```python
from build123d import *

# Parameters (mm, degrees)
SKETCH_W        = 130
SKETCH_H        = 200
PAD_DEPTH       = 2.5
SKETCH001_R     = 2.5
POCKET_DEPTH    = 5.001
SKETCH002_W     = 10
SKETCH002_H     = 5
POCKET001_DEPTH = 5.001
SKETCH003_W     = 5
SKETCH003_H     = 10
PAD001_DEPTH    = 5
SKETCH004_W     = 10
SKETCH004_H     = 5
PAD002_DEPTH    = 5
FILLET_R        = 7


with BuildPart() as part:
    # Sketch → Pad (new body, symmetric)
    with BuildSketch(Plane.YZ):
        Rectangle(SKETCH_W, SKETCH_H)
    extrude(amount=PAD_DEPTH, both=True)

    # Sketch001 (on Face6 of Pad) → Pocket (cut, through all)
    with BuildSketch(Plane.YZ.offset(2.5)):
        with Locations((-45, -20)):
            Circle(SKETCH001_R)
        with Locations((50, -20)):
            Circle(SKETCH001_R)
    extrude(amount=-POCKET_DEPTH, mode=Mode.SUBTRACT)

    # Sketch002 (on Face5 of Pocket) → Pocket001 (cut, through all)
    with BuildSketch(Plane.YZ.offset(2.5)):
        with Locations((-60, -87.5)):
            Rectangle(SKETCH002_W, SKETCH002_H)
        with Locations((-40, -87.5)):
            Rectangle(SKETCH002_W, SKETCH002_H)
        with Locations((-20, -87.5)):
            Rectangle(SKETCH002_W, SKETCH002_H)
        with Locations((0, -87.5)):
            Rectangle(SKETCH002_W, SKETCH002_H)
        with Locations((20, -87.5)):
            Rectangle(SKETCH002_W, SKETCH002_H)
        with Locations((40, -87.5)):
            Rectangle(SKETCH002_W, SKETCH002_H)
        with Locations((60, -87.5)):
            Rectangle(SKETCH002_W, SKETCH002_H)
    extrude(amount=-POCKET001_DEPTH, mode=Mode.SUBTRACT)

    # Sketch003 (on Face5 of Pocket001) → Pad001 (join)
    with BuildSketch(Plane.YZ.offset(2.5)):
        with Locations((67.5, 95)):
            Rectangle(SKETCH003_W, SKETCH003_H)
        with Locations((67.5, 75)):
            Rectangle(SKETCH003_W, SKETCH003_H)
        with Locations((67.5, 55)):
            Rectangle(SKETCH003_W, SKETCH003_H)
        with Locations((67.5, 35)):
            Rectangle(SKETCH003_W, SKETCH003_H)
        with Locations((67.5, 15)):
            Rectangle(SKETCH003_W, SKETCH003_H)
        with Locations((67.5, -5)):
            Rectangle(SKETCH003_W, SKETCH003_H)
        with Locations((67.5, -25)):
            Rectangle(SKETCH003_W, SKETCH003_H)
        with Locations((67.5, -45)):
            Rectangle(SKETCH003_W, SKETCH003_H)
        with Locations((67.5, -65)):
            Rectangle(SKETCH003_W, SKETCH003_H)
    extrude(amount=-PAD001_DEPTH)

    # Sketch004 (on Face69 of Pad001) → Pad002 (join)
    with BuildSketch(Plane.YZ.offset(2.5)):
        with Locations((32.5, 102.5)):
            Rectangle(SKETCH004_W, SKETCH004_H)
        with Locations((52.5, 102.5)):
            Rectangle(SKETCH004_W, SKETCH004_H)
    extrude(amount=-PAD002_DEPTH)

    # Fillet
    fillet_edges = [part.edges().sort_by_distance(p)[0] for p in [
        (0, -65, 100),
    ]]
    fillet(fillet_edges, radius=FILLET_R)


solid = part.part
```
The model under review builds one solid part; all positions refer to its coordinate system, in mm. A direction names the side the tool comes from. Round coordinates to 2 decimals unless told otherwise and drop trailing zeros. Loops run counter-clockwise (first coordinate to the right, second up) from the corner with the lowest first, then second, coordinate; pieces in that order, holes last. Notation, with made-up numbers: M -35,-12.75 L -30,-12.75 A8 cw -30,-4.75 Z; hole C 27,59.25 d4. An arc over 180 degrees is marked long. Put each result on its own line as item: value.
Q1. Consider section D-D, the plane z = -36.5. Give the boundary of the cut face in (x, y), then the cut area to 3 significant figures.
Result set:
outline: M -2.5,-65 L 2.5,-65 L 2.5,65 L -2.5,65 Z
area: 650 mm²
Q2. For pin 1 (2.5 mm diameter, centred on x = 0.5, y = 59, fed in from +Z); pin 2 (1.5 mm diameter, centred on x = -0.5, y = -61.5, fed in from +Z); pin 3 (2.5 mm diameter, centred on x = 0.5, z = -88.5, fed in from -Y), all flat-tipped, find the tip position at first contact; note any pin that passes through.
Result set:
pin 1: stops at z = 100
pin 2: stops at z = 99.44
pin 3: stops at y = -55
Q3. Machinability: for faces 1 (the flat face through (0, -40, -85)), 2 (the flat face through (0, 57.5, 102)), 3 (the flat face through (0, 60, -90)), 4 (the flat face through (0, -55, -88)), which of the approach directions +Z, -Z, +X, -X, +Y, -Y give a long, thin tool a straight path to every point of the face, cutting with its end or side? Answer none if there is none.
Result set:
face 1: +X, -X
face 2: +Z, +X, -X, +Y
face 3: +X, -X, +Y
face 4: +X, -X, -Y
Q4. Mouldability with a two-part tool opening along Z and no side actions: class faces 5 (the flat face through (0, 65, -55)), 6 (the flat face through (0, -16, 100)), 7 (the flat face through (0, 67, 40)), 8 (the flat face through (2.5, 2, 4)) as released by +Z, released by -Z, zero draft, split by the parting line, or undercut.
Result set:
face 5: undercut
face 6: released by +Z
face 7: undercut
face 8: zero draft
Q5. To check wall thickness, follow L1, parallel to Z at x = -0.6, y = 40.5; L2, parallel to Y at x = -0.1, z = -21.5; L3, parallel to Y at x = -0.4, z = 83. State the ranges of each line that lie inside material, in increasing order.
Result set:
L1: z = -100 to -90, -85 to 100
L2: y = -65 to -47, -43 to 48, 52 to 70
L3: y = -65 to 65
Q6. Consider section A-A, the plane y = 50. Give the boundary of the cut face in (x, z).
Result set:
outline: M -2.5,-100 L 2.5,-100 L 2.5,-22.5 L -2.5,-22.5 Z; M -2.5,-17.5 L 2.5,-17.5 L 2.5,105 L -2.5,105 Z
Q7. Consider section C-C, the plane y = -2. Give the boundary of the cut face in (x, z).
Result set:
outline: M -2.5,-100 L 2.5,-100 L 2.5,-90 L -2.5,-90 Z; M -2.5,-85 L 2.5,-85 L 2.5,100 L -2.5,100 Z
Q8. Consider section B-B, the plane x = 1.75. Count the separate pieces of the cut face and the enclosed holes in it, then the cut area to 3 significant figures.
Result set:
separate pieces: 1
enclosed holes: 7
area: 26,200 mm²
